```python
from build123d import *

# Parameters (mm, degrees)
F0_W     = 73
F0_H     = 78
F0_W_2   = 112
F0_H_2   = 35
F1_DEPTH = 5
F2_R     = 5
F3_R     = 5
F6_D     = 4.1
F8_D     = 43
F9_D     = 11


# Not quite as in the source:
# - a feature names something its author has since deleted; it is built from what else it names


with BuildPart() as f1:
    # F0 (on Top) → F1 (new body)
    with BuildSketch(Plane.XY):
        Polygon((-56, 50), (-86, 50), (-272.5, -15), (-272.5, -50), (-199.5, -50), (199.5, -50), (272.5, -50), (272.5, -15), (86, 50), (56, 50), align=None)
        with Locations((-236, -89)):
            Rectangle(F0_W, F0_H)
        with Locations((236, -89)):
            Rectangle(F0_W, F0_H)
        with Locations((0, 67.5)):
            Rectangle(F0_W_2, F0_H_2)
    extrude(amount=F1_DEPTH)

    # F2
    f2_edges = [f1.edges().sort_by_distance(p)[0] for p in [
        (-272.5, -128, 2.5),
        (-199.5, -128, 2.5),
        (199.5, -128, 2.5),
        (272.5, -128, 2.5),
        (272.5, -15, 2.5),
        (-272.5, -15, 2.5),
        (-199.5, -50, 2.5),
        (199.5, -50, 2.5),
        (-56, 50, 2.5),
        (-56, 85, 2.5),
        (56, 85, 2.5),
        (56, 50, 2.5),
    ]]
    fillet(f2_edges, radius=F2_R)

    # F3
    f3_edges = [f1.edges().sort_by_distance(p)[0] for p in [
        (86, 50, 2.5),
        (-86, 50, 2.5),
    ]]
    fillet(f3_edges, radius=F3_R)

    # F6 (through all)
    with Locations(Plane(origin=(0, 0, 0), x_dir=(1, 0, 0), z_dir=(0, 0, -1))):
        with Locations((-31, -17.5), (31, -17.5)):
            Hole(F6_D / 2)

    # F8 (through all)
    with Locations(Plane(origin=(0, 0, 0), x_dir=(1, 0, 0), z_dir=(0, 0, -1))):
        with Locations((-236, 94), (236, 94)):
            Hole(F8_D / 2)

    # F9 (through all)
    with Locations(Plane(origin=(0, 0, 0), x_dir=(1, 0, 0), z_dir=(0, 0, -1))):
        with Locations((-20.5, -68.5), (20.5, -68.5), (-20.5, 33.5), (20.5, 33.5)):
            Hole(F9_D / 2)


solid = f1.part
```
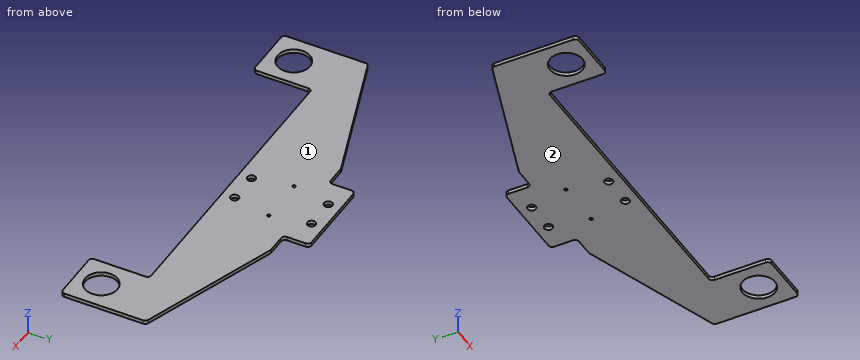
The model under review builds one solid part; all positions refer to its coordinate system, in mm. Face numbers are marked on the shaded views. Give positions to 0.01 mm unless a question says otherwise; leave off trailing zeros. Write each loop counter-clockwise with the first axis right and the second up, starting at its lowest first coordinate (ties: lowest second). Pieces come first, ordered by that corner, then holes. Notation, with made-up numbers: (57.5, 86.5) - (66.5, 86.5) arc R29 ccw to (66.5, 109.5) - close; hole circle Ø8 at (59.5, -15). An arc over 180 degrees is marked (long way). Answer in a Markdown table with one row per item. Add a question column.
1. We need section A-A on y = -33.5. Write out the cut boundary in (x, z), then the cut area to 4 significant figures.
2. We need section B-B on x = 20.5. Write out the cut boundary in (y, z), then the cut area to 3 significant figures.
3. We need section C-C on x = -236. Write out the cut boundary in (y, z).
4. We need section D-D on z = 1.2. State how many separate pieces and enclosed holes the cut face has, then the cut area to 3 significant figures.
5. Insertion check: P1, Ø3.5, axis at x = 31, y = 17.5, coming from the +Z side; P2, Ø3, axis at x = 93.5, z = 4, coming from the -Y side. Each pin has a flat end and moves straight along its axis. Give the tip position at first contact, or say it passes through.
6. Wall thickness on line 1 along X through (y, z) = (-33.5, 2.7); line 2 along Y through (x, z) = (-20.5, 2.9); line 3 along X through (y, z) = (68.5, 1.3): over which ranges is each line inside the solid? List them lowest first. Write a range as [from, to].
7. Draft analysis for pull direction Z (two halves, no side actions). For the marked faces 1 and 2, state which applies: +Z half, -Z half, draft (parallel to the pull), parting line (faces both ways), or undercut.
Ans:
| question | item | result |
|---|---|---|
| 1 | outline | (-272.5, 0) - (-26, 0) - (-26, 5) - (-272.5, 5) - close; (-15, 0) - (15, 0) - (15, 5) - (-15, 5) - close; (26, 0) - (272.5, 0) - (272.5, 5) - (26, 5) - close |
| 1 | area | 2,615 mm^2 |
| 2 | outline | (-50, 0) - (-39, 0) - (-39, 5) - (-50, 5) - close; (-28, 0) - (63, 0) - (63, 5) - (-28, 5) - close; (74, 0) - (85, 0) - (85, 5) - (74, 5) - close |
| 2 | area | 565 mm^2 |
| 3 | outline | (-128, 0) - (-115.5, 0) - (-115.5, 5) - (-128, 5) - close; (-72.5, 0) - (-2.28, 0) - (-2.28, 5) - (-72.5, 5) - close |
| 4 | separate pieces | 1 |
| 4 | enclosed holes | 8 |
| 4 | area | 54,400 mm^2 |
| 5 | P1 | passes through |
| 5 | P2 | stops at y = -50 |
| 6 | line 1 | x = [-272.5, -26], [-15, 15], [26, 272.5] |
| 6 | line 2 | y = [-50, -39], [-28, 63], [74, 85] |
| 6 | line 3 | x = [-56, -26], [-15, 15], [26, 56] |
| 7 | face 1 | +Z half |
| 7 | face 2 | -Z half |
